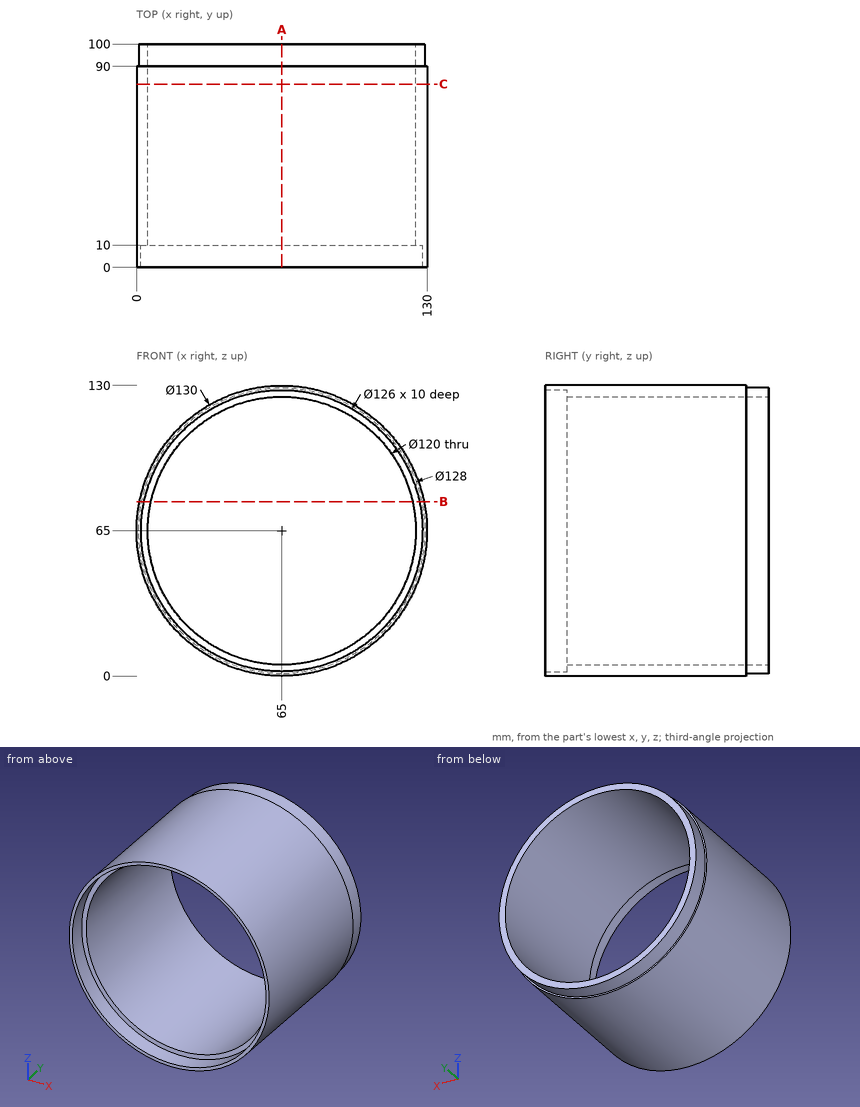
Input: dimensioned drawing with shaded views. Units: mm. Origin: part minimum x, y, z. Coordinates: 2 decimals unless noted, no trailing zeros. Loops run counter-clockwise (first coordinate to the right, second up) from the corner with the lowest first, then second, coordinate; pieces in that order, holes last. Notation, with made-up numbers: (89.5, 37) -> (148.5, 37) arc R12 ccw to (148.5, 50) -> close; hole circle Ø1 at (-29, 63.5). An arc over 180 degrees is marked (long way). Use a Markdown table: item, result. Add a question column.
(1) Line query: line 1 along X through (y, z) = (38.5, 65); line 2 along Y through (x, z) = (5.5, 51); line 3 along X through (y, z) = (3.25, 65). Output: solid intervals per line, ascending.
(2) Section query A-A, the plane x = 65. Return loops of the section in (y, z).
(3) Pin query (flat end, axial travel): pin 1 Ø8 at (x, y) = (111.5, 64) entering from +Z; pin 2 Ø12 at (x, y) = (37, 58) entering from +Z; pin 3 Ø8 at (y, z) = (17.5, 83) entering from +X. Return the tip coordinate at first contact, or that it passes through.
(4) Section query C-C, the plane y = 82. Return loops of the section in (x, z).
(5) Section query B-B, the plane z = 78. Return loops of the section in (x, y).
Answer:
| question | item | result |
|---|---|---|
| 1 | line 1 | x = 0 to 5, 125 to 130 |
| 1 | line 2 | y = 10 to 100 |
| 1 | line 3 | x = 0 to 2, 128 to 130 |
| 2 | outline | (0, 0) -> (90, 0) -> (90, 1) -> (100, 1) -> (100, 5) -> (10, 5) -> (10, 2) -> (0, 2) -> close; (0, 128) -> (10, 128) -> (10, 125) -> (100, 125) -> (100, 129) -> (90, 129) -> (90, 130) -> (0, 130) -> close |
| 3 | pin 1 | stops at z = 114.18 |
| 3 | pin 2 | stops at z = 126.16 |
| 3 | pin 3 | stops at x = 128.47 |
| 4 | outline | circle Ø130 at (65, 65); hole circle Ø120 at (65, 65) |
| 5 | outline | (1.31, 0) -> (3.36, 0) -> (3.36, 10) -> (6.43, 10) -> (6.43, 100) -> (2.33, 100) -> (2.33, 90) -> (1.31, 90) -> close; (123.57, 10) -> (126.64, 10) -> (126.64, 0) -> (128.69, 0) -> (128.69, 90) -> (127.67, 90) -> (127.67, 100) -> (123.57, 100) -> close |
